The listing builds one solid part. Answer for the finished solid, in the listing's coordinates (mm). A direction names the side the tool comes from. Coordinates: 2 decimals unless noted, no trailing zeros. Write each loop counter-clockwise with the first axis right and the second up, starting at its lowest first coordinate (ties: lowest second). Pieces come first, ordered by that corner, then holes.
```python
from build123d import *

# Parameters (mm, degrees)
EXTRUDE_1_DEPTH     = 5
SKETCH_4_W          = 40
SKETCH_4_H          = 8.5
CUT_EXTRUDE_1_DEPTH = 5
SKETCH_5_R          = 1.2
CUT_EXTRUDE_2_DEPTH = 7
SKETCH_9_R          = 9
CUT_EXTRUDE_3_DEPTH = 1.5
SKETCH_10_R         = 3
SKETCH_10_R_2       = 0.6
CUT_EXTRUDE_4_DEPTH = 5
SKETCH_11_R         = 2.25
CUT_EXTRUDE_5_DEPTH = 1


with BuildPart() as part:
    # 草图3 → 凸台-拉伸1 (new body)
    with BuildSketch(Plane.XY):
        with BuildLine():
            Line((-35.723215038, 7.743839121), (-58.858024221, -11.158625231))
            ThreePointArc((-58.858024221, -11.158625231), (-60.178030432, -31.612892204), (-39.681768347, -31.462245799))
            Line((-39.681768347, -31.462245799), (-22.972363252, -13.241253001))
            ThreePointArc((-22.972363252, -13.241253001), (-19.627898346, -10.846108205), (-15.602197786, -10))
            Line((-15.602197786, -10), (15.602197786, -10))
            ThreePointArc((15.602197786, -10), (19.627898346, -10.846108205), (22.972363252, -13.241253001))
            Line((22.972363252, -13.241253001), (39.681768347, -31.462245799))
            ThreePointArc((39.681768347, -31.462245799), (60.178030432, -31.612892204), (58.858024221, -11.158625231))
            Line((58.858024221, -11.158625231), (35.723215038, 7.743839121))
            ThreePointArc((35.723215038, 7.743839121), (32.754745755, 9.419086771), (29.39605488, 10))
            Line((29.39605488, 10), (-29.39605488, 10))
            ThreePointArc((-29.39605488, 10), (-32.754745755, 9.419086771), (-35.723215038, 7.743839121))
        make_face()
    extrude(amount=EXTRUDE_1_DEPTH)

    # 草图4 → 切除-拉伸1 (cut)
    with BuildSketch(Plane.XY.offset(5)):
        with Locations((0, -0.75)):
            Rectangle(SKETCH_4_W, SKETCH_4_H)
    extrude(amount=-CUT_EXTRUDE_1_DEPTH, mode=Mode.SUBTRACT)

    # 草图5 → 切除-拉伸2 (cut)
    with BuildSketch(Plane.XY.offset(5)):
        with Locations((-29, -5)):
            Circle(SKETCH_5_R)
        with Locations((-29, 5)):
            Circle(SKETCH_5_R)
    cut_extrude_2 = extrude(amount=-CUT_EXTRUDE_2_DEPTH, mode=Mode.SUBTRACT)

    # 镜向1: 切除-拉伸2 across plane
    add(cut_extrude_2.mirror(Plane.ZY), mode=Mode.SUBTRACT)

    # 草图9 → 切除-拉伸3 (cut)
    with BuildSketch(Plane(origin=(0, 0, 0), x_dir=(-1, 0, 0), z_dir=(0, 0, -1))):
        with Locations((-50, -22)):
            Circle(SKETCH_9_R)
    cut_extrude_3 = extrude(amount=-CUT_EXTRUDE_3_DEPTH, mode=Mode.SUBTRACT)

    # 草图10 → 切除-拉伸4 (cut)
    with BuildSketch(Plane(origin=(0, 0, 1.5), x_dir=(-1, 0, 0), z_dir=(0, 0, -1))):
        with Locations((-50, -22)):
            Circle(SKETCH_10_R)
        with Locations((-57.5, -22)):
            Circle(SKETCH_10_R_2)
        with Locations((-42.5, -22)):
            Circle(SKETCH_10_R_2)
    cut_extrude_4 = extrude(amount=-CUT_EXTRUDE_4_DEPTH, mode=Mode.SUBTRACT)

    # 镜向3: 切除-拉伸3, 切除-拉伸4 across plane
    add(cut_extrude_3.mirror(Plane.ZY), mode=Mode.SUBTRACT)
    add(cut_extrude_4.mirror(Plane.ZY), mode=Mode.SUBTRACT)

    # 草图11 → 切除-拉伸5 (cut)
    with BuildSketch(Plane.XY.offset(5)):
        with Locations((-57.5, -22)):
            Circle(SKETCH_11_R)
        with Locations((-42.5, -22)):
            Circle(SKETCH_11_R)
    cut_extrude_5 = extrude(amount=-CUT_EXTRUDE_5_DEPTH, mode=Mode.SUBTRACT)

    # 镜向4: 切除-拉伸5 across plane
    add(cut_extrude_5.mirror(Plane.ZY), mode=Mode.SUBTRACT)


solid = part.part
```
(1) Find the intervals of material crossed by probe 1 along X at (y, z) = (-4, 1.9); probe 2 along Y at (x, z) = (-11.5, 1.9); probe 3 along X at (y, z) = (-14, 1.2), in increasing order.
(2) For a pull along Y with two mould halves and no side action, classify faces 4 (the cylindrical face through (-42.988, -24.196, 4.507)), 5 (the cylindrical face through (-19.68, -10.87, 2.46)), 6 (the cylindrical face through (32.8, 9.403, 2.465)) as pulls with the +Y half, pulls with the -Y half, needs draft (parallel to the pull), parting line crosses it, or undercut.
(3) Each of these flat-tipped pins is pushed along its axis until it touches: pin 1 (9.5 mm diameter, centred on x = 50, y = -22, fed in from +Z); pin 2 (1.4 mm diameter, centred on x = -57.5, y = -22, fed in from +Z); pin 3 (1 mm diameter, centred on x = 42.5, z = 1, fed in from +Y); pin 4 (16 mm diameter, centred on x = -50, y = -22, fed in from -Z). Where does it stop, or does it pass through?
(4) Section B-B, the plane y = -27.5 is taken. Write down the section's boundary in (x, z), plus the area to 3 significant figures.
(5) Section C-C, the plane y = 5 is taken. Write down the section's boundary in (x, z).
(6) Which of the six approach directions +Z, -Z, +X, -X, +Y, -Y give full straight-line access (tool end or side, diameter ignored) to faces 1 (the flat face through (57, -21, 4)), 2 (the cylindrical face through (19.57, -10.82, 2.46)), 3 (the flat face through (0, 3.5, 3))?
(7) Section A-A, the plane x = -1 is taken. Write down the section's boundary in (y, z), plus the area to 3 significant figures.
(8) Section D-D, the plane x = 50 is taken. Write down the section's boundary in (y, z), plus the area to 3 significant figures.
Solution:
1. probe 1: x = -50.1 to -29.66, -28.34 to -20, 20 to 28.34, 29.66 to 50.1
1. probe 2: y = -10 to -5, 3.5 to 10
1. probe 3: x = -61.49 to -54.12, -45.88 to -23.67, 23.67 to 45.88, 54.12 to 61.49
2. face 4: undercut
2. face 5: pulls with the -Y half
2. face 6: pulls with the +Y half
3. pin 1: stops at z = 5
3. pin 2: stops at z = 4
3. pin 3: stops at y = 2.62
3. pin 4: stops at z = 1.5
4. outline: (-62.87, 0) - (-57.12, 0) - (-57.12, 1.5) - (-42.88, 1.5) - (-42.88, 0) - (-36.05, 0) - (-36.05, 5) - (-62.87, 5) - close; (36.05, 0) - (42.88, 0) - (42.88, 1.5) - (57.12, 1.5) - (57.12, 0) - (62.87, 0) - (62.87, 5) - (36.05, 5) - close
4. area: 226 mm2
5. outline: (-39.08, 0) - (-30.2, 0) - (-30.2, 5) - (-39.08, 5) - close; (-27.8, 0) - (27.8, 0) - (27.8, 5) - (-27.8, 5) - close; (30.2, 0) - (39.08, 0) - (39.08, 5) - (30.2, 5) - close
6. face 1: +Z
6. face 2: +Z, -Z, -Y
6. face 3: +Z, -Z
7. outline: (-10, 0) - (-5, 0) - (-5, 5) - (-10, 5) - close; (3.5, 0) - (10, 0) - (10, 5) - (3.5, 5) - close
7. area: 57.5 mm2
8. outline: (-36, 0) - (-31, 0) - (-31, 1.5) - (-25, 1.5) - (-25, 5) - (-36, 5) - close; (-19, 1.5) - (-13, 1.5) - (-13, 0) - (-3.92, 0) - (-3.92, 5) - (-19, 5) - close
8. area: 112 mm2
